from build123d import *

# Parameters (mm, degrees)
F0_R     = 101.5
F1_DEPTH = 15
F2_R     = 88.5
F3_DEPTH = 15.001
F4_T     = -2


# Not quite as in the source:
# - a feature names something its author has since deleted; it is built from what else it names


with BuildPart() as f1:
    # F0 (on Top) → F1 (new body)
    with BuildSketch(Plane.XY):
        Circle(F0_R)
    extrude(amount=F1_DEPTH)

    # F2 (on face) → F3 (cut, through all)
    with BuildSketch(Plane.XY.offset(15)):
        Circle(F2_R)
    extrude(amount=-F3_DEPTH, mode=Mode.SUBTRACT)

    # F4
    f4_openings = [f1.faces().sort_by_distance(p)[0] for p in [
        (-98.629146, 0, 15),
    ]]
    offset(amount=F4_T, openings=f4_openings)


solid = f1.part
Source: CAD feature listing. Evaluate the final solid. Frame: model axes, mm. A direction names the side the tool comes from. Give positions to 0.01 mm unless a question says otherwise; leave off trailing zeros. Write each loop counter-clockwise with the first axis right and the second up, starting at its lowest first coordinate (ties: lowest second). Pieces come first, ordered by that corner, then holes. Notation, with made-up numbers: M 61.25,13.25 L 115.25,13.25 A25 cw 115.25,30.25 Z; hole C 72.25,32.5 d4. An arc over 180 degrees is marked long. Return JSON: item names as keys, results as strings. Group by question number.
1) Material intervals for line 1 along Y through (x, z) = (0, 6.25); line 2 along Y through (x, z) = (-2.5, 1.75); line 3 along X through (y, z) = (63, 13), sorted ascending. Write a range as [from, to].
2) Cut plane A-A, the plane x = 0. Output: boundary loops of the cut face in (y, z), plus the area to 3 significant figures.
3) Pull-direction query (X, two-part tool) for faces 1 (the face through (22, -88, 2)), 2 (the face through (7, 91, 0)), 3 (the face through (96.813, 30.488, 7.395)); classes: pulls with the +X half, pulls with the -X half, needs draft (parallel to the pull), parting line crosses it, or undercut.
4) Pin query (flat end, axial travel): P1, Ø2, axis at x = 9, z = 3, coming from the -Y side; P2, Ø3, axis at x = -65.5, z = 9.5, coming from the +Y side; P3, Ø5, axis at y = -41.5, z = 5.5, coming from the +X side. Return the tip coordinate at first contact, or that it passes through.
5) Cut plane C-C, the plane z = 8.5. Output: boundary loops of the cut face in (x, y).
6) Set-up query: faces 4 (the face through (86.32, 27.18, 8.59)), 5 (the face through (-19.185, -86.396, 7.605)). Return all of +Z, -Z, +X, -X, +Y, -Y with unobstructed straight access to the full face (end or side cutting, diameter ignored); none if empty.
Recorded:
{
 "1": {"line 1": "y = [-101.5, -99.5], [-90.5, -88.5], [88.5, 90.5], [99.5, 101.5]", "line 2": "y = [-101.47, -88.46], [88.46, 101.47]", "line 3": "x = [-79.58, -77.01], [-64.97, -62.16], [62.16, 64.97], [77.01, 79.58]"},
 "2": {"outline": "M -101.5,0 L -88.5,0 L -88.5,15 L -90.5,15 L -90.5,2 L -99.5,2 L -99.5,15 L -101.5,15 Z; M 88.5,0 L 101.5,0 L 101.5,15 L 99.5,15 L 99.5,2 L 90.5,2 L 90.5,15 L 88.5,15 Z", "area": "156 mm²"},
 "3": {"face 1": "undercut", "face 2": "needs draft", "face 3": "parting line crosses it"},
 "4": {"P1": "stops at y = -101.18", "P2": "stops at y = 78.78", "P3": "stops at x = 93.71"},
 "5": {"outline": "C 0,0 d203; C 0,0 d181; hole C 0,0 d199; hole C 0,0 d177"},
 "6": {"face 4": "+Z", "face 5": "+Z, -Z"}
}
